from build123d import *

# Parameters (mm, degrees)
SKETCH_1_R      = 4
EXTRUDE_1_DEPTH = 60
SKETCH_2_R      = 6
EXTRUDE_2_DEPTH = 2
EXTRUDE_START   = 6.2
SKETCH_3_R      = 4
EXTRUDE_3_DEPTH = 6.2
SKETCH_4_R      = 6
EXTRUDE_4_DEPTH = 2


with BuildPart() as part:
    # Эскиз1 → Бобышка-Вытянуть1 (new, symmetric)
    with BuildSketch(Plane.XY):
        Circle(SKETCH_1_R)
    extrude(amount=EXTRUDE_1_DEPTH, both=True)

    # Эскиз2 → Бобышка-Вытянуть2 (add)
    with BuildSketch(Plane.XY.offset(60)):
        Circle(SKETCH_2_R)
    extrude_2 = extrude(amount=EXTRUDE_2_DEPTH)

    # Эскиз3 → Бобышка-Вытянуть3 (add)
    with BuildSketch(Plane.XY.offset(62).offset(EXTRUDE_START)):
        Circle(SKETCH_3_R)
    extrude_3 = extrude(amount=-EXTRUDE_3_DEPTH)

    # Эскиз4 → Бобышка-Вытянуть4 (add)
    with BuildSketch(Plane.XY.offset(68.2)):
        Circle(SKETCH_4_R)
    extrude_4 = extrude(amount=EXTRUDE_4_DEPTH)

    # Зеркальное отражение1: Бобышка-Вытянуть2, Бобышка-Вытянуть3, Бобышка-Вытянуть4 across plane
    add(extrude_2.mirror(Plane.XY))
    add(extrude_3.mirror(Plane.XY))
    add(extrude_4.mirror(Plane.XY))


solid = part.part
Input: part model. Units: mm. Frame: model coordinates. A direction names the side the tool comes from. Coordinates: 2 decimals unless noted, no trailing zeros. Loops run counter-clockwise (first coordinate to the right, second up) from the corner with the lowest first, then second, coordinate; pieces in that order, holes last.
Q1. Draft query along Z for faces 3 (the face through (-1.42, -3.92, -62)), 4 (the face through (0, 0, -70.2)), 5 (the face through (-6, 0, 61)). Return one class per face: +Z half, -Z half, draft (parallel to the pull), parting line (faces both ways), or undercut.
Q2. Cut plane A-A (x = 0). Output: boundary loops of the cut face in (y, z), then the cut area to 3 significant figures.
Q3. Cut plane C-C (z = -30.5). Output: boundary loops of the cut face in (x, y), then the cut area to 3 significant figures.
Q4. Set-up query: faces 1 (the face through (-0.867, -3.905, -65.143)), 2 (the face through (-6, 0, -61)). Return all of +Z, -Z, +X, -X, +Y, -Y with unobstructed straight access to the full face (end or side cutting, diameter ignored); none if empty.
Q5. Material intervals for line 1 (Z direction, x = -4, y = -2.25); line 2 (X direction, y = -2.75, z = -4); line 3 (X direction, y = -2, z = 48), sorted ascending.
Q6. Contact query for flat-ended pins moving along their axis: pin 1 (3 mm diameter, centred on x = -3, z = 49, fed in from -Y); pin 2 (4 mm diameter, centred on y = -3.5, z = -0.5, fed in from -X); pin 3 (6 mm diameter, centred on x = -5, z = -48, fed in from -Y). Output: stop coordinate, or through.
Working result:
1. face 3: undercut
1. face 4: -Z half
1. face 5: draft
2. outline: (-6, -70.2) - (6, -70.2) - (6, -68.2) - (4, -68.2) - (4, -62) - (6, -62) - (6, -60) - (4, -60) - (4, 60) - (6, 60) - (6, 62) - (4, 62) - (4, 68.2) - (6, 68.2) - (6, 70.2) - (-6, 70.2) - (-6, 68.2) - (-4, 68.2) - (-4, 62) - (-6, 62) - (-6, 60) - (-4, 60) - (-4, -60) - (-6, -60) - (-6, -62) - (-4, -62) - (-4, -68.2) - (-6, -68.2) - close
2. area: 1,160 mm2
3. outline: circle Ø8 at (0, 0)
3. area: 50.3 mm2
4. face 1: none
4. face 2: +Z, -Z
5. line 1: z = -70.2 to -68.2, -62 to -60, 60 to 62, 68.2 to 70.2
5. line 2: x = -2.9 to 2.9
5. line 3: x = -3.46 to 3.46
6. pin 1: stops at y = -3.71
6. pin 2: stops at x = -3.71
6. pin 3: stops at y = -3.46
